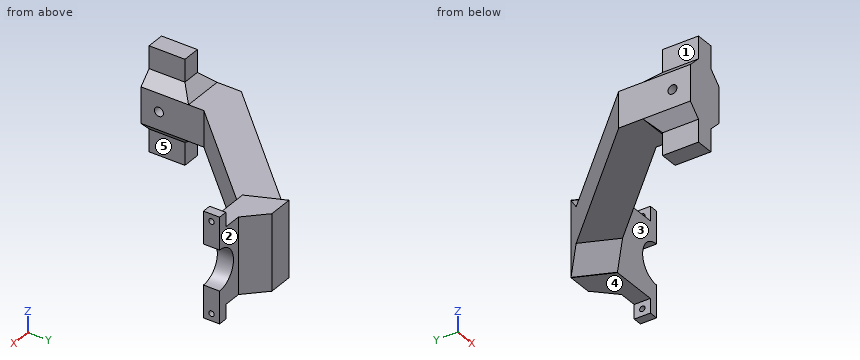
from build123d import *

# Parameters (mm, degrees)
BOSS_EXTRUDE1_DEPTH      = 25.4
BOSS_EXTRUDE4_DEPTH      = 24.13
BOSS_EXTRUDE4_DEPTH_BACK = 49.53
SKETCH7_W                = 12.7
SKETCH7_H                = 25.4
SKETCH8_R                = 3.175
CUT_EXTRUDE3_DEPTH       = 219.535967291
CHAMFER3_SIZE            = 8.255
BOSS_EXTRUDE5_DEPTH      = 14.224
BOSS_EXTRUDE5_DEPTH_BACK = 39.624
SKETCH9_R                = 14.224
CUT_EXTRUDE4_DEPTH       = 188.728167838
SKETCH11_W               = 33.274
SKETCH11_H               = 53.848
CUT_EXTRUDE5_DEPTH       = 13.97
CHAMFER4_SIZE            = 13.97
CHAMFER5_SIZE            = 13.97
SKETCH18_W               = 6.35
SKETCH18_H               = 11.43
BOSS_EXTRUDE6_DEPTH      = 10.16
SKETCH19_W               = 6.35
SKETCH19_H               = 11.43
BOSS_EXTRUDE7_DEPTH      = 10.16
SKETCH20_R               = 1.905
CUT_EXTRUDE7_DEPTH       = 10.16


with BuildPart() as part:
    # Sketch2 → Boss-Extrude1 (new body)
    with BuildSketch(Plane.XY):
        Polygon((0, 0), (50.8, 0), (50.8, -25.4), (10.806439585, -25.4), (-68.58, -107.87941775), (-68.58, -152.4), (-97.79, -152.4), (-97.79, -101.6), align=None)
    extrude(amount=BOSS_EXTRUDE1_DEPTH)

    # Sketch7 → Boss-Extrude4 (add, two sides: drawn at the far end of the back side and taken through both)
    with BuildSketch(Plane.XY.offset(25.4).offset(-BOSS_EXTRUDE4_DEPTH_BACK)):
        with Locations((-83.185, -139.7)):
            Rectangle(SKETCH7_W, SKETCH7_H)
    extrude(amount=BOSS_EXTRUDE4_DEPTH + BOSS_EXTRUDE4_DEPTH_BACK)

    # Sketch8 → Cut-Extrude3 (cut, through all)
    with BuildSketch(Plane.ZY.offset(97.79)):
        with Locations((12.7, -139.7)):
            Circle(SKETCH8_R)
    extrude(amount=-CUT_EXTRUDE3_DEPTH, mode=Mode.SUBTRACT)

    # Chamfer3
    chamfer3_edges = [part.edges().sort_by_distance(p)[0] for p in [
        (-76.835, -139.7, 25.4),
        (-76.835, -139.7, 0),
        (-83.185, -127, 25.4),
        (-83.185, -127, 0),
        (-89.535, -139.7, 25.4),
        (-89.535, -139.7, 0),
    ]]
    chamfer(chamfer3_edges, length=CHAMFER3_SIZE - 0.0001)  # a hair under: the kernel refuses the full size

    # Sketch10 → Boss-Extrude5 (add, two sides: drawn at the far end of the back side and taken through both)
    with BuildSketch(Plane.XY.offset(25.4).offset(-BOSS_EXTRUDE5_DEPTH_BACK)):
        Polygon((0, 0), (10.806439585, -25.4), (50.8, -25.4), (50.8, 0), align=None)
    extrude(amount=BOSS_EXTRUDE5_DEPTH + BOSS_EXTRUDE5_DEPTH_BACK)

    # Sketch9 → Cut-Extrude4 (cut, through all)
    with BuildSketch(Plane(origin=(0, 0, 0), x_dir=(1, 0, 0), z_dir=(0, 1, 0))):
        with Locations((50.8, -12.7)):
            Circle(SKETCH9_R)
    extrude(amount=-CUT_EXTRUDE4_DEPTH, mode=Mode.SUBTRACT)

    # Sketch11 → Cut-Extrude5 (cut)
    with BuildSketch(Plane(origin=(0, 0, 0), x_dir=(1, 0, 0), z_dir=(0, 1, 0))):
        with Locations((34.163, -12.7)):
            Rectangle(SKETCH11_W, SKETCH11_H)
    extrude(amount=-CUT_EXTRUDE5_DEPTH, mode=Mode.SUBTRACT)

    # Chamfer4
    chamfer4_edges = [part.edges().sort_by_distance(p)[0] for p in [
        (17.526, -13.97, 12.7),
    ]]
    chamfer(chamfer4_edges, length=CHAMFER4_SIZE - 0.0001)  # a hair under: the kernel refuses the full size

    # Chamfer5
    chamfer5_edges = [part.edges().sort_by_distance(p)[0] for p in [
        (5.403219792, -12.7, 0),
        (5.403219792, -12.7, 25.4),
    ]]
    chamfer(chamfer5_edges, length=CHAMFER5_SIZE)

    # Sketch18 → Boss-Extrude6 (add)
    with BuildSketch(Plane.XY.offset(39.624)):
        with Locations((47.625, -19.685)):
            Rectangle(SKETCH18_W, SKETCH18_H)
    extrude(amount=BOSS_EXTRUDE6_DEPTH)

    # Sketch19 → Boss-Extrude7 (add)
    with BuildSketch(Plane(origin=(0, 0, -14.224), x_dir=(-1, 0, 0), z_dir=(0, 0, -1))):
        with Locations((-47.625, -19.685)):
            Rectangle(SKETCH19_W, SKETCH19_H)
    extrude(amount=BOSS_EXTRUDE7_DEPTH)

    # Sketch20 → Cut-Extrude7 (cut)
    with BuildSketch(Plane(origin=(50.8, 0, 0), x_dir=(0, 0, -1), z_dir=(1, 0, 0))):
        with Locations((-44.704, -19.685)):
            Circle(SKETCH20_R)
        with Locations((19.304, -19.685)):
            Circle(SKETCH20_R)
    extrude(amount=-CUT_EXTRUDE7_DEPTH, mode=Mode.SUBTRACT)


solid = part.part
Could you check a few things on this model? Use its own coordinates, in mm. Face numbers are marked on the shaded views. A direction names the side the tool comes from. Give positions to 0.01 mm unless a question says otherwise; leave off trailing zeros. Order: outer loops, then holes, each group sorted by start corner. A loop starts at its lowest first (then second) coordinate and runs counter-clockwise, first axis right, second up. Notation, with made-up numbers: (19, 24.5) - (71, 24.5) arc R14 ccw to (71, 29.5) - close; hole circle Ø11 at (63.25, 37). An arc over 180 degrees is marked (long way). One line per question, with ' | ' between items. Start each with the question number.
Item 1: I want a section at D-D on x = -41. Write out the boundary of the cut face in (y, z).
Item 2: I need wall thicknesses on probe 1 along Z at (x, y) = (-86.5, -139.7) (3 decimals); probe 2 along X at (y, z) = (-142.5, 41) (3 decimals); probe 3 along Z at (x, y) = (-81, -131). Which ranges of each line are inside material? Lowest first, please. Write a range as [from, to].
Item 3: I'm going to push flat-ended pins straight in: pin 1 Ø9.5 at (x, z) = (41.5, 9) entering from +Y; pin 2 Ø6 at (y, z) = (-19.685, -19.304) entering from +X; pin 3 Ø6.5 at (x, y) = (-85, -138) entering from -Z; pin 4 Ø12.5 at (y, z) = (-139, 38) entering from -X. Where does each tip first touch, or does it pass through?
Item 4: For the marked faces 1, 2, 3, 4 and 5, which set-ups out of +Z, -Z, +X, -X, +Y, -Y let a thin tool reach every point of the face, with its end or its side?
Verdict:
1) outline: (-79.22, 0) - (-42.6, 0) - (-42.6, 25.4) - (-79.22, 25.4) - close
2) probe 1: [-24.13, 9.525], [15.875, 49.53] | probe 2: [-89.535, -76.835] | probe 3: [-24.13, 49.53]
3) pin 1: y = -13.97 | pin 2: x = 50.8 | pin 3: z = -24.13 | pin 4: x = -91.44
4) face 1: +Z, -X, +Y, -Y | face 2: +Z, -Z, +X, +Y | face 3: +Z, -Z, +X, -Y | face 4: -Z, -X, +Y, -Y | face 5: -Z, +X, +Y, -Y
